from build123d import *

# Parameters (mm, degrees)
F0_R     = 50
F0_R_2   = 42.5
F1_DEPTH = 15
F2_SIZE2 = 7.49999
F2_SIZE  = 14.99999
F3_R     = 3.5


# Not quite as in the source:
# - a fillet or chamfer is up to 0.001 mm smaller than in the source, because OpenCascade refuses the exact size


with BuildPart() as f1:
    # F0 (on Top) → F1 (new body, symmetric)
    with BuildSketch(Plane.XY):
        Circle(F0_R)
        Circle(F0_R_2, mode=Mode.SUBTRACT)
    extrude(amount=F1_DEPTH, both=True)

    # F2 (size 15 and 7.5 in the source; OpenCascade refuses exactly that, so slightly less here)
    f2_edges = [f1.edges().sort_by_distance(p)[0] for p in [
        (-50, 0, -15),
    ]]
    f2_side = f1.faces().sort_by_distance((-50, 0, 0))[0]
    chamfer(f2_edges, length=F2_SIZE, length2=F2_SIZE2, reference=f2_side)

    # F3
    f3_edges = [f1.edges().sort_by_distance(p)[0] for p in [
        (-50, 0, 15),
        (-42.5, 0, 15),
    ]]
    fillet(f3_edges, radius=F3_R)


solid = f1.part
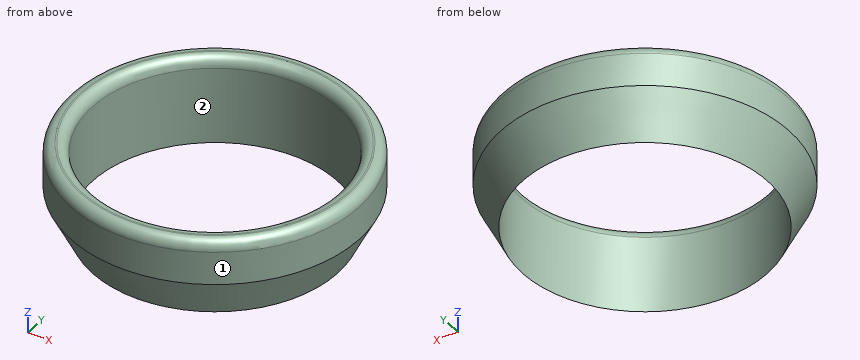
Input: part model. Units: mm. Frame: model coordinates. Face numbers are marked on the shaded views. Coordinates: 2 decimals unless noted, no trailing zeros. Loops run counter-clockwise (first coordinate to the right, second up) from the corner with the lowest first, then second, coordinate; pieces in that order, holes last. Notation, with made-up numbers: (27, -3.75) -> (42, -3.75) arc R9 cw to (42, 3.25) -> close; hole circle Ø5 at (3.5, 29). An arc over 180 degrees is marked (long way). Write item = value, one per line. Start each with the question number.
Item 1: Cut plane D-D, the plane z = 6.5. Return loops of the section in (x, y), plus the area to 3 significant figures.
Item 2: First-contact query: P1, Ø6, axis at x = -21.5, z = 3.5, coming from the +Y side; P2, Ø4, axis at x = 16, z = 6.5, coming from the +Y side; P3, Ø6, axis at y = -5, z = 0, coming from the +X side. Flat tips, straight axial feed; report the tip coordinate or a pass-through.
Item 3: Material intervals for line 1 (Y direction, x = 0, z = 3.75); line 2 (Y direction, x = -12.5, z = -7); line 3 (X direction, y = 36.5, z = -7.75), sorted ascending.
Item 4: Mould query, pull axis Y, two halves, no side actions, for the marked faces 1 and 2. Classes: pulls with the +Y half, pulls with the -Y half, needs draft (parallel to the pull), parting line crosses it, or undercut.
Ans:
q1.outline = circle Ø100 at (0, 0); hole circle Ø85 at (0, 0)
q1.area = 2,180 mm²
q2.P1 = 46.45
q2.P2 = 48
q2.P3 = 49.96
q3.line_1 = -50 to -42.5, 42.5 to 50
q3.line_2 = -44.79 to -40.62, 40.62 to 44.79
q3.line_3 = -28.2 to -21.77, 21.77 to 28.2
q4.face_1 = parting line crosses it
q4.face_2 = undercut
